from build123d import *

# Parameters (mm, degrees)
IZIM1_R                     = 13.5
IZIM1_R_2                   = 5.1
IZIM1_R_3                   = 18
IZIM1_R_4                   = 7
Y_KSEKLIK_EKSTR_ZYON1_DEPTH = 10


with BuildPart() as part:
    # Çizim1 → Yükseklik-Ekstrüzyon1 (new body)
    with BuildSketch(Plane(origin=(0, 0, 0), x_dir=(0, 0, -1), z_dir=(1, 0, 0))):
        Polygon((-250, 350), (-250, 570), (0, 570), (0, 350), (500, 0), (500, -200), (500, -240), (-250, -240), (-250, -200), align=None)
        with Locations((-203.812062632, 211.374016696)):
            Circle(IZIM1_R, mode=Mode.SUBTRACT)
        with Locations((-183.812062632, 231.374016696)):
            Circle(IZIM1_R_2, mode=Mode.SUBTRACT)
        with Locations((-223.812062632, 231.374016696)):
            Circle(IZIM1_R_2, mode=Mode.SUBTRACT)
        with Locations((-183.812062632, 191.374016696)):
            Circle(IZIM1_R_2, mode=Mode.SUBTRACT)
        with Locations((-223.812062632, 191.374016696)):
            Circle(IZIM1_R_2, mode=Mode.SUBTRACT)
        Circle(IZIM1_R_3, mode=Mode.SUBTRACT)
        with Locations((-38.890872965, 38.890872965)):
            Circle(IZIM1_R_2, mode=Mode.SUBTRACT)
        with Locations((38.890872965, 38.890872965)):
            Circle(IZIM1_R_2, mode=Mode.SUBTRACT)
        with Locations((38.890872965, -38.890872965)):
            Circle(IZIM1_R_2, mode=Mode.SUBTRACT)
        with Locations((-38.890872965, -38.890872965)):
            Circle(IZIM1_R_2, mode=Mode.SUBTRACT)
        with Locations((-210, 550)):
            Circle(IZIM1_R_4, mode=Mode.SUBTRACT)
        with Locations((-153.333333333, 550)):
            Circle(IZIM1_R_4, mode=Mode.SUBTRACT)
        with Locations((-96.666666667, 550)):
            Circle(IZIM1_R_4, mode=Mode.SUBTRACT)
        with Locations((-40, 550)):
            Circle(IZIM1_R_4, mode=Mode.SUBTRACT)
        with Locations((-210, -220)):
            Circle(IZIM1_R_4, mode=Mode.SUBTRACT)
        with Locations((-114.285714286, -220)):
            Circle(IZIM1_R_4, mode=Mode.SUBTRACT)
        with Locations((-18.571428571, -220)):
            Circle(IZIM1_R_4, mode=Mode.SUBTRACT)
        with Locations((77.142857143, -220)):
            Circle(IZIM1_R_4, mode=Mode.SUBTRACT)
        with Locations((172.857142857, -220)):
            Circle(IZIM1_R_4, mode=Mode.SUBTRACT)
        with Locations((268.571428571, -220)):
            Circle(IZIM1_R_4, mode=Mode.SUBTRACT)
        with Locations((364.285714286, -220)):
            Circle(IZIM1_R_4, mode=Mode.SUBTRACT)
        with Locations((460, -220)):
            Circle(IZIM1_R_4, mode=Mode.SUBTRACT)
        Polygon((29.246579563, 281.988117893), (0, 240.207289947), (9.011551126, 233.899204159), (38.258130688, 275.680032105), align=None, mode=Mode.SUBTRACT)
        Polygon((-200.681608906, 45.789510008), (-220.902149255, 81.456437938), (-230.471325041, 76.031414918), (-210.250784693, 40.364486987), align=None, mode=Mode.SUBTRACT)
    extrude(amount=Y_KSEKLIK_EKSTR_ZYON1_DEPTH)


solid = part.part
Part model, mm, in its own coordinate system. A direction names the side the tool comes from. Coordinates: 2 decimals unless noted, no trailing zeros. Loops run counter-clockwise (first coordinate to the right, second up) from the corner with the lowest first, then second, coordinate; pieces in that order, holes last. Notation, with made-up numbers: (-0.75, 32) - (14.25, 32) arc R15 cw to (14.25, 53) - close; hole circle Ø6 at (82.25, 44.5). An arc over 180 degrees is marked (long way). Write each question's results on one line, items separated by ' | '. Start each with the question number.
Q1. Drop flat-ended pins along their axis: pin 1 Ø18 at (y, z) = (-220, -364.29) entering from -X; pin 2 Ø5 at (x, z) = (4, -37) entering from +Y; pin 3 Ø8 at (y, z) = (-38.89, -38.89) entering from +X; pin 4 Ø1.5 at (x, z) = (4, -150.5) entering from +Y (3 decimals). Give the stop position or say it passes through.
Q2. Which spindle directions (+Z, -Z, +X, -X, +Y, -Y) get a long thin tool onto all of the face, cutting with end or side? Do faces 1 (the flat face through (10, 81, -47)), 2 (the flat face through (4.93, 254.5, -23.43)). Say none if no direction does.
Q3. Slice it at C-C on x = 8. Give the number of separate pieces and of enclosed holes in the cut face, and give its area (3 significant figures).
Q4. Slice it at B-B on y = 380. Give the cut face in (x, z).
Q5. Probe line 1 along Z through (x, y) = (5.25, 550); line 2 along Y through (x, z) = (0.75, 213); line 3 along Z through (x, y) = (1, 478). List the from-to ranges inside material, lowest first.
Q6. Two-plate mould, pull along Z, no slides. Class faces 3 (the flat face through (4.93, 177.45, -246.5)), 4 (the cylindrical face through (4.93, 17.847, 2.343)), 5 (the flat face through (4.93, 261.39, -14.83)), 6 (the flat face through (0, 81, -47)): +Z half, -Z half, draft (parallel to the pull), parting line (faces both ways), or undercut.
Q7. Slice it at A-A on z = -193. Give the cut face in (x, y), and give its area (3 significant figures).
Answer:
1) pin 1: stops at x = 0 | pin 2: stops at y = 325.85 | pin 3: passes through | pin 4: stops at y = 245.175
2) face 1: +Z, -Z, +X, +Y, -Y | face 2: +X, -X
3) separate pieces: 1 | enclosed holes: 24 | area: 405,000 mm2
4) outline: (0, 0) - (10, 0) - (10, 250) - (0, 250) - close
5) line 1: z = 0 to 33, 47 to 89.67, 103.67 to 146.33, 160.33 to 203, 217 to 250 | line 2: y = -240 to -226.32, -213.68 to 45.21, 67.52 to 201.48, 221.27 to 543.68, 556.32 to 570 | line 3: z = 0 to 250
6) face 3: -Z half | face 4: undercut | face 5: undercut | face 6: draft
7) outline: (0, -240) - (10, -240) - (10, 214.9) - (0, 214.9) - close | area: 4,550 mm2
